```python
from build123d import *

# Parameters (mm, degrees)
F0_W     = 203.2
F0_H     = 127
F1_DEPTH = 127
F3_DEPTH = 76.2
F4_SIZE2 = 101.6
F4_SIZE  = 76.2
F5_R     = 5.08
F6_R     = 15.24
F7_DEPTH = 50.801
F8_R     = 17.78
F9_DEPTH = 127.001


with BuildPart() as f1:
    # F0 (on Front) → F1 (new body)
    with BuildSketch(Plane.XZ):
        Rectangle(F0_W, F0_H)
    extrude(amount=F1_DEPTH)

    # F2 (on face) → F3 (cut)
    with BuildSketch(Plane.XZ.offset(127)):
        Polygon((-38.1, 0), (-38.1, -63.5), (101.6, -63.5), (101.6, 63.5), (0, 63.5), (0, 0), align=None)
    extrude(amount=-F3_DEPTH, mode=Mode.SUBTRACT)

    # F4
    f4_edges = [f1.edges().sort_by_distance(p)[0] for p in [
        (101.6, -25.4, 63.5),
    ]]
    f4_side = f1.faces().sort_by_distance((-21.771429, -52.614286, 63.5))[0]
    chamfer(f4_edges, length=F4_SIZE, length2=F4_SIZE2, reference=f4_side)

    # F5
    f5_edges = [f1.edges().sort_by_distance(p)[0] for p in [
        (0, -127, 31.75),
        (-19.05, -127, 0),
        (-38.1, -127, -31.75),
        (-69.85, -127, -63.5),
        (-101.6, -127, 0),
        (-50.8, -127, 63.5),
        (0, -88.9, 63.5),
        (0, -88.9, 0),
        (0, -50.8, 31.75),
        (-38.1, -88.9, 0),
        (-38.1, -88.9, -63.5),
        (-38.1, -50.8, -31.75),
        (-38.1, 0, 63.5),
        (25.4, -25.4, 63.5),
        (-101.6, -63.5, 63.5),
        (12.7, -50.8, 63.5),
        (-101.6, -63.5, -63.5),
        (-101.6, 0, 0),
        (0, 0, -63.5),
        (31.75, -50.8, -63.5),
        (-19.05, -50.8, 0),
    ]]
    fillet(f5_edges, radius=F5_R)

    # F6 (on face) → F7 (cut, through all)
    with BuildSketch(Plane.XZ.offset(50.8)):
        with Locations((17.78, -17.78)):
            Circle(F6_R)
    extrude(amount=-F7_DEPTH, mode=Mode.SUBTRACT)

    # F8 (on face) → F9 (cut, through all)
    with BuildSketch(Plane.XY.offset(63.5)):
        with Locations((-75.203537941, -57.9331703484)):
            Circle(F8_R)
    extrude(amount=-F9_DEPTH, mode=Mode.SUBTRACT)


solid = f1.part
```
Design review of the part built by this model. Coordinates are the model's own, in mm. A direction names the side the tool comes from. Round coordinates to 2 decimals unless told otherwise and drop trailing zeros. Write each loop counter-clockwise with the first axis right and the second up, starting at its lowest first coordinate (ties: lowest second). Pieces come first, ordered by that corner, then holes. Notation, with made-up numbers: (7.5, 34.25) -> (45.5, 34.25) arc R17 cw to (45.5, 42.25) -> close; hole circle Ø1 at (-11.75, 26.25). An arc over 180 degrees is marked (long way). Answer in a Markdown table with one row per item.
Q1. To check wall thickness, follow L1, parallel to Z at x = 17.78, y = -30.5; L2, parallel to Y at x = -74.5, z = -41; L3, parallel to Z at x = -32, y = -84. State the ranges of each line that lie inside material, in increasing order. Write a range as [from, to].
The answers:
| item | result |
|---|---|
| L1 | [-63.5, -33.02], [-2.54, 63.5] |
| L2 | [-127, -75.7], [-40.17, 0] |
| L3 | [0, 63.5] |
Q2. Clearance check with flat-ended pins moving along their axes: pin 1 Ø8.5 at (x, y) = (-21, -86.5) entering from -Z; pin 2 Ø3 at (y, z) = (-43.5, -21.5) entering from +X (3 decimals); pin 3 Ø3 at (x, z) = (2, 49.5) entering from -Y. State where each tip first meets the part, or that it passes through.
The answers:
| item | result |
|---|---|
| pin 1 | z = 0 |
| pin 2 | x = 90.275 |
| pin 3 | y = -53.68 |
Q3. Take a section at B-B, the plane z = -15. State the section outline as (x, y) points (3 decimals), then the cut area to 3 significant figures.
The answers:
| item | result |
|---|---|
| outline | (-101.6, -121.92) arc R5.08 ccw to (-96.52, -127) -> (-43.18, -127) arc R5.08 ccw to (-38.1, -121.92) -> (-38.1, -55.88) arc R5.08 cw to (-33.02, -50.8) -> (2.796, -50.8) -> (2.796, 0) -> (-96.52, 0) arc R5.08 ccw to (-101.6, -5.08) -> close; (32.764, -50.8) -> (84.275, -50.8) -> (84.275, 0) -> (32.764, 0) -> close; hole circle Ø35.56 at (-75.204, -57.933) |
| area | 11,800 mm² |
Q4. Draft analysis for pull direction X (two halves, no side actions). For faces 1 (the face through (-1.528, -88.438, 62.051)), 2 (the face through (-19.246, -125.551, 1.528)), 3 (the face through (-79.06, -75.29, 0.89)), 4 (the face through (5.686, -25.756, -27.053)), state which applies: +X half, -X half, draft (parallel to the pull), parting line (faces both ways), or undercut.
The answers:
| item | result |
|---|---|
| face 1 | +X half |
| face 2 | draft |
| face 3 | undercut |
| face 4 | undercut |
Q5. Take a section at C-C, the plane y = -103.5. State the section outline as (x, z) points.
The answers:
| item | result |
|---|---|
| outline | (-101.6, -58.42) arc R5.08 ccw to (-96.52, -63.5) -> (-43.18, -63.5) arc R5.08 ccw to (-38.1, -58.42) -> (-38.1, -5.08) arc R5.08 cw to (-33.02, 0) -> (-5.08, 0) arc R5.08 ccw to (0, 5.08) -> (0, 58.42) arc R5.08 ccw to (-5.08, 63.5) -> (-96.52, 63.5) arc R5.08 ccw to (-101.6, 58.42) -> close |
Q6. Take a section at A-A, the plane x = 17.78. State the section outline as (y, z) points, then the cut area to 3 significant figures.
The answers:
| item | result |
|---|---|
| outline | (-50.8, -58.42) arc R5.08 ccw to (-45.72, -63.5) -> (-5.08, -63.5) arc R5.08 ccw to (0, -58.42) -> (0, -33.02) -> (-50.8, -33.02) -> close; (-50.8, -2.54) -> (0, -2.54) -> (0, 58.42) arc R5.08 ccw to (-5.08, 63.5) -> (-45.72, 63.5) arc R5.08 ccw to (-50.8, 58.42) -> close |
| area | 4,880 mm² |
Q7. For faces 5 (the face through (-32.775, -1.528, 62.051)), 6 (the face through (-1.449, -88.438, 1.528)), 7 (the face through (0, -89, 32)), list the 3-axis set-ups (+Z, -Z, +X, -X, +Y, -Y) from which the entire face can be reached by the end or side of a thin tool; tool diameter is ignored.
The answers:
| item | result |
|---|---|
| face 5 | +Z, +X, -X, +Y |
| face 6 | -Z, +X, -Y |
| face 7 | +Z, -Z, +X, -Y |
Q8. Take a section at D-D, the plane z = 52. State the section outline as (x, y) points (3 decimals).
The answers:
| item | result |
|---|---|
| outline | (-101.6, -121.92) arc R5.08 ccw to (-96.52, -127) -> (-5.08, -127) arc R5.08 ccw to (0, -121.92) -> (0, -55.88) arc R5.08 cw to (5.08, -50.8) -> (34.025, -50.8) -> (34.025, 0) -> (-96.52, 0) arc R5.08 ccw to (-101.6, -5.08) -> close; hole circle Ø35.56 at (-75.204, -57.933) |
